```python
from build123d import *

# Parameters (mm, degrees)
BOSS_EXTRUDE1_START  = -17
BOSS_EXTRUDE1_DEPTH  = 35
SKETCH2_R            = 10.45
CUT_EXTRUDE1_DEPTH   = 32
SKETCH3_R            = 6.5
CUT_EXTRUDE2_DEPTH   = 62.814237842
SKETCH4_R            = 12.5
CUT_EXTRUDE3_DEPTH   = 64.419239983
FILLET5_R            = 10
FILLET6_R            = 10
FILLET5_OF_MIRROR1_R = 10
FILLET6_OF_MIRROR1_R = 10


with BuildPart() as part:
    # Sketch1 → Boss-Extrude1 (new body)
    with BuildSketch(Plane.YZ.offset(BOSS_EXTRUDE1_START)):
        with BuildLine():
            Line((-14, 0), (-14, 51))
            Line((-14, 51), (14, 51))
            Line((14, 51), (14, 0))
            ThreePointArc((14, 0), (0, -14), (-14, 0))
        make_face()
    boss_extrude1 = extrude(amount=BOSS_EXTRUDE1_DEPTH)

    # Sketch2 → Cut-Extrude1 (cut)
    with BuildSketch(Plane.YZ.offset(18)):
        with Locations(Location((0, 0, 0), (0, 0, 270))):
            Circle(SKETCH2_R)
    cut_extrude1 = extrude(amount=-CUT_EXTRUDE1_DEPTH, mode=Mode.SUBTRACT)

    # Sketch3 → Cut-Extrude2 (cut, through all)
    with BuildSketch(Plane.YZ.offset(-14)):
        with Locations(Location((0, 0, 0), (0, 0, 270))):
            Circle(SKETCH3_R)
    cut_extrude2 = extrude(amount=-CUT_EXTRUDE2_DEPTH, mode=Mode.SUBTRACT)

    # Sketch4 → Cut-Extrude3 (cut, through all)
    with BuildSketch(Plane.YZ.offset(18)):
        with Locations(Location((0, 35.95, 0), (0, 0, 270))):
            Circle(SKETCH4_R)
    cut_extrude3 = extrude(amount=-CUT_EXTRUDE3_DEPTH, mode=Mode.SUBTRACT)

    # Fillet5
    fillet5_edges = [part.edges().sort_by_distance(p)[0] for p in [
        (0.5, 14, 51),
    ]]
    fillet(fillet5_edges, radius=FILLET5_R)

    # Fillet6
    fillet6_edges = [part.edges().sort_by_distance(p)[0] for p in [
        (0.5, -14, 51),
    ]]
    fillet(fillet6_edges, radius=FILLET6_R)

    # Mirror1: Boss-Extrude1, Cut-Extrude1, Cut-Extrude2, Cut-Extrude3 across plane
    add(boss_extrude1.mirror(Plane.XY))
    add(cut_extrude1.mirror(Plane.XY), mode=Mode.SUBTRACT)
    add(cut_extrude2.mirror(Plane.XY), mode=Mode.SUBTRACT)
    add(cut_extrude3.mirror(Plane.XY), mode=Mode.SUBTRACT)

    # Fillet5 of Mirror1
    fillet5_of_mirror1_edges = [part.edges().sort_by_distance(p)[0] for p in [
        (0.5, 14, -51),
    ]]
    fillet(fillet5_of_mirror1_edges, radius=FILLET5_OF_MIRROR1_R)

    # Fillet6 of Mirror1
    fillet6_of_mirror1_edges = [part.edges().sort_by_distance(p)[0] for p in [
        (0.5, -14, -51),
    ]]
    fillet(fillet6_of_mirror1_edges, radius=FILLET6_OF_MIRROR1_R)


solid = part.part
```
Verification items for the finished model (mm, model axes). Coordinates: 2 decimals unless noted, no trailing zeros. Loops run counter-clockwise (first coordinate to the right, second up) from the corner with the lowest first, then second, coordinate; pieces in that order, holes last. Notation, with made-up numbers: (87.5, 51.5) -> (94.5, 51.5) arc R27 cw to (94.5, 89.5) -> close; hole circle Ø5 at (42, -22). An arc over 180 degrees is marked (long way). Answer in a Markdown table with one row per item.
1) Scan lines: line 1 along Y through (x, z) = (-2.5, 0); line 2 along Z through (x, y) = (16.5, -11.25); line 3 along Y through (x, z) = (-15, 0). Record each from-to range of solid material in increasing order. Write a range as from..to.
The answers:
| item | result |
|---|---|
| line 1 | y = -14..-10.45, 10.45..14 |
| line 2 | z = -47.89..-41.4, -30.5..30.5, 41.4..47.89 |
| line 3 | y = -14..-6.5, 6.5..14 |
2) Depth check by flat-ended pin: P1, Ø3, axis at x = 4, y = -6, coming from the +Z side. Enter the tip coordinate at first touch or a pass-through.
The answers:
| item | result |
|---|---|
| P1 | stops at z = 50.99 |
3) Section check C-C (y = 9.5). Record the cut outline in (x, z).
The answers:
| item | result |
|---|---|
| outline | (-17, -49.35) -> (18, -49.35) -> (18, -44.07) -> (-17, -44.07) -> close; (-17, -27.83) -> (18, -27.83) -> (18, -4.35) -> (-14, -4.35) -> (-14, 4.35) -> (18, 4.35) -> (18, 27.83) -> (-17, 27.83) -> close; (-17, 44.07) -> (18, 44.07) -> (18, 49.35) -> (-17, 49.35) -> close |
4) Section check D-D (y = -5). Record the cut outline in (x, z).
The answers:
| item | result |
|---|---|
| outline | (-17, -50.95) -> (18, -50.95) -> (18, -47.41) -> (-17, -47.41) -> close; (-17, -24.49) -> (18, -24.49) -> (18, -9.18) -> (-14, -9.18) -> (-14, -4.15) -> (-17, -4.15) -> close; (-17, 4.15) -> (-14, 4.15) -> (-14, 9.18) -> (18, 9.18) -> (18, 24.49) -> (-17, 24.49) -> close; (-17, 47.41) -> (18, 47.41) -> (18, 50.95) -> (-17, 50.95) -> close |
5) Section check A-A (x = 15). Record the cut outline in (y, z), and give its area (3 significant figures).
The answers:
| item | result |
|---|---|
| outline | (-14, -41) arc R10 ccw to (-4, -51) -> (4, -51) arc R10 ccw to (14, -41) -> (14, 41) arc R10 ccw to (4, 51) -> (-4, 51) arc R10 ccw to (-14, 41) -> close; hole circle Ø25 at (0, -35.95); hole circle Ø25 at (0, 35.95); hole circle Ø20.9 at (0, 0) |
| area | 1,450 mm2 |
6) Section check B-B (z = 35.95). Record the cut outline in (x, y), and give its area (3 significant figures).
The answers:
| item | result |
|---|---|
| outline | (-17, -14) -> (18, -14) -> (18, -12.5) -> (-17, -12.5) -> close; (-17, 12.5) -> (18, 12.5) -> (18, 14) -> (-17, 14) -> close |
| area | 105 mm2 |
7) Draft check along Z on faces 1 (the face through (0, 0, 51)), 2 (the face through (2.224, 3.139, 9.967)), 3 (the face through (0, 0, -51)), 4 (the face through (-14, 0, 7)). Enter one of: released by +Z, released by -Z, zero draft, split by the parting line, or undercut.
The answers:
| item | result |
|---|---|
| face 1 | released by +Z |
| face 2 | undercut |
| face 3 | released by -Z |
| face 4 | undercut |
